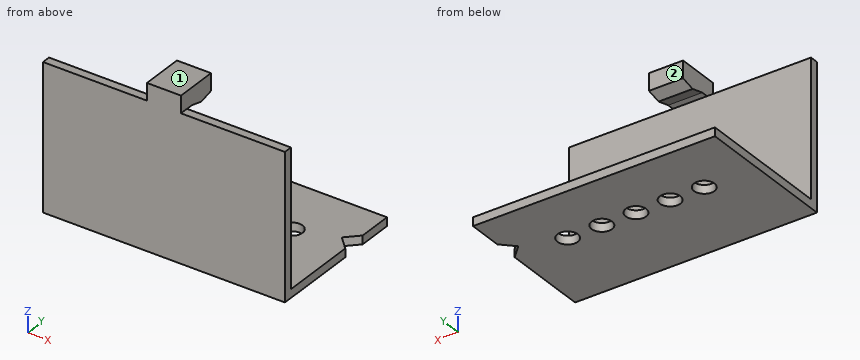
Autodesk Inventor part; units mm, degrees
ref_plane "YZ Plane" through (0, 0, 0) normal (1, 0, 0) x (0, 1, 0)
ref_plane "XZ Plane" through (0, 0, 0) normal (0, 1, 0) x (-1, 0, 0)
ref_plane "XY Plane" through (0, 0, 0) normal (0, 0, 1) x (1, 0, 0)
sketch "Sketch1" plane through (0, 0, 0) normal (0, 1, 0) x (-1, 0, 0)
  line L0 (45.085, 26.9875) -> (-45.085, 26.9875)
  line L1 (-45.085, 26.9875) -> (-45.085, -26.9875)
  line L2 (-45.085, -26.9875) -> (45.085, -26.9875)
  line L3 (45.085, -26.9875) -> (45.085, 26.9875)
  point P0 (0, 0)
  dimension "d0" = 90.17
  dimension "d1" = 45.085
  dimension "d2" = 53.975
  dimension "d3" = 26.9875
extrude "Extrusion1" add sketch "Sketch1" along normal blind 53.975
sketch "Sketch2" plane through (45.085, 0, 26.9875) normal (1, 0, 0) x (0, 0, -1)
  line L0 (0, 53.975) -> (53.975, 53.975)
  line L1 (0, 53.975) -> (50.8, 53.975)
  line L2 (50.8, 53.975) -> (50.8, 3.175)
  line L3 (50.8, 3.175) -> (0, 3.175)
  line L4 (0, 3.175) -> (0, 53.975)
  line L5 (0, 0) -> (53.975, 0)
  line L6 (53.975, 0) -> (53.975, 53.975)
  point P0 (26.9875, 0)
  dimension "d6" = 3.175
  dimension "d7" = 3.175
extrude "Extrusion2" cut sketch "Sketch2" against normal through all
sketch "Sketch3" plane through (0, 0, 0) normal (0, -1, 0) x (1, 0, 0)
  line L0 (-6.35, 23.8125) -> (6.35, 23.8125)
  line L1 (6.35, 23.8125) -> (6.35, 33.3375)
  line L2 (6.35, 33.3375) -> (-6.35, 33.3375)
  line L3 (-6.35, 33.3375) -> (-6.35, 23.8125)
  line L4 (1.9102, 23.8125) -> (1.9102, 26.9875) construction
  line L5 (-45.085, 26.9875) -> (45.085, 26.9875)
  point P0 (0, 0)
  dimension "d10" = 12.7
  dimension "d11" = 9.525
  dimension "d12" = 3.175
  dimension "d13" = 6.35
extrude "Extrusion3" add sketch "Sketch3" against normal blind 15.875
sketch "Sketch4" plane through (6.35, 0, 33.3375) normal (1, 0, 0) x (0, 0, -1)
  line L0 (9.525, 3.175) -> (6.35, 3.175)
  line L1 (9.525, 3.175) -> (9.525, 15.875)
  line L2 (0, 15.875) -> (9.525, 15.875)
  line L3 (6.35, 0) -> (6.35, 3.175)
  line L4 (6.35, 3.175) -> (6.35, 5.715)
  line L5 (6.35, 5.715) -> (6.35, 15.875) construction
  line L6 (6.35, 5.715) -> (7.62, 10.795)
  line L7 (7.62, 10.795) -> (6.35, 15.875)
  point P0 (33.3375, 0)
  dimension "d19" = 1.27
  dimension "d20" = 10.16
extrude "Extrusion4" cut sketch "Sketch4" against normal blind 15.875
sketch "Sketch5" plane through (45.085, 0, -26.9875) normal (0, 0, -1) x (-1, 0, 0)
  line L0 (19.6342, 31.75) -> (32.3596, 31.75) construction
  line L1 (32.3596, 31.75) -> (45.085, 31.75) construction
  line L2 (45.085, 31.75) -> (57.8104, 31.75) construction
  line L3 (57.8104, 31.75) -> (70.5358, 31.75) construction
  circle A0 centre (19.6342, 31.75) radius 3.81
  circle A1 centre (32.3596, 31.75) radius 3.81
  circle A2 centre (45.085, 31.75) radius 3.81
  circle A3 centre (57.8104, 31.75) radius 3.81
  circle A4 centre (70.5358, 31.75) radius 3.81
  line L4 (19.6342, 31.75) -> (5.2747, 31.75) construction
  line L5 (70.5358, 31.75) -> (84.8953, 31.75) construction
  line L6 (0, 53.975) -> (90.17, 53.975)
  point P0 (45.085, 0)
  point P1 (86.995, 3.175)
  point P2 (3.175, 3.175)
  dimension "d23" = 12.7254
  dimension "d24" = 7.62
  dimension "d26" = 22.225
extrude "Extrusion5" cut sketch "Sketch5" against normal blind 15.875
sketch "Sketch6" plane through (45.085, 3.175, -23.8125) normal (0, 0, 1) x (1, 0, 0)
  line L0 (0, 37.8968) -> (-4.572, 33.3248)
  line L1 (-4.572, 33.3248) -> (0, 28.7528)
  line L2 (0, 50.8) -> (-90.17, 50.8)
  line L3 (0, 37.8968) -> (0, 50.8)
  line L4 (0, 28.7528) -> (0, 25.3386)
  line L5 (0, 50.8) -> (0, 0)
  point P0 (-45.085, -3.175)
  dimension "d31" = 12.9032
  dimension "d32" = 45
  dimension "d33" = 45
  dimension "d35" = 4.572
extrude "Extrusion6" cut sketch "Sketch6" against normal blind 25.4
properties part number "PCB_Case02B"
For this review, take the finished solid that the model builds, in its own axes (mm). Face numbers are marked on the shaded views. A direction names the side the tool comes from. Round coordinates to 2 decimals unless told otherwise and drop trailing zeros. Order: outer loops, then holes, each group sorted by start corner. A loop starts at its lowest first (then second) coordinate and runs counter-clockwise, first axis right, second up. Notation, with made-up numbers: M 76,42.5 L 115,42.5 A29 cw 115,72.5 Z; hole C 9.5,68 d7. An arc over 180 degrees is marked long. Use a Markdown table: item, result. Add a question column.
Item 1: To check wall thickness, follow line 1 along X through (y, z) = (31, -25) (3 decimals); line 2 along Y through (x, z) = (0, -25.5) (3 decimals); line 3 along Z through (x, y) = (-11.5, 7). State the ranges of each line that lie inside material, in increasing order.
Item 2: Add section D-D, the plane z = 29. Give the boundary of the cut face in (x, y) (3 decimals), then the cut area to 3 significant figures.
Item 3: Insertion check: pin 1 (12 mm diameter, centred on x = 14, z = -18, fed in from +Y) (3 decimals); pin 2 (2 mm diameter, centred on x = -3.5, y = 20, fed in from +Z); pin 3 (6 mm diameter, centred on x = 12.73, y = 31.75, fed in from +Z) (3 decimals); pin 4 (4 mm diameter, centred on y = 5, z = 29, fed in from -X). Each pin has a flat end and moves straight along its axis. Give the tip position at first contact, or say it passes through.
Item 4: Add section B-B, the plane x = 0. Give the boundary of the cut face in (y, z) (1 decimal), then the cut area to 3 significant figures.
Item 5: Add section C-C, the plane y = 29.5. Give the boundary of the cut face in (x, z) (1 decimal).
Item 6: Tool access review of the marked faces 1 and 2: name each direction out of +Z, -Z, +X, -X, +Y, -Y from which nothing blocks a thin tool from reaching the whole face with its end or side.
Geometry results:
| question | item | result |
|---|---|---|
| 1 | line 1 | x = -45.085 to -29.186, -21.715 to -16.461, -8.99 to -3.735, 3.735 to 8.99, 16.461 to 21.715, 29.186 to 45.085 |
| 1 | line 2 | y = 0 to 27.94, 35.56 to 53.975 |
| 1 | line 3 | z = -26.99 to -23.81 |
| 2 | outline | M -6.35,0 L 6.35,0 L 6.35,15.875 L -6.35,15.875 Z |
| 2 | area | 202 mm² |
| 3 | pin 1 | stops at y = 53.975 |
| 3 | pin 2 | stops at z = -23.81 |
| 3 | pin 3 | passes through |
| 3 | pin 4 | stops at x = -6.35 |
| 4 | outline | M 0,-27 L 27.9,-27 L 27.9,-23.8 L 3.2,-23.8 L 3.2,27 L 5.7,27 L 10.8,25.7 L 15.9,27 L 15.9,33.3 L 0,33.3 Z; M 35.6,-27 L 54,-27 L 54,-23.8 L 35.6,-23.8 Z |
| 4 | area | 416 mm² |
| 5 | outline | M -45.1,-27 L -28.5,-27 L -28.5,-23.8 L -45.1,-23.8 Z; M -22.4,-27 L -15.8,-27 L -15.8,-23.8 L -22.4,-23.8 Z; M -9.7,-27 L -3.1,-27 L -3.1,-23.8 L -9.7,-23.8 Z; M 3.1,-27 L 9.7,-27 L 9.7,-23.8 L 3.1,-23.8 Z; M 15.8,-27 L 22.4,-27 L 22.4,-23.8 L 15.8,-23.8 Z; M 28.5,-27 L 45.1,-27 L 45.1,-23.8 L 28.5,-23.8 Z |
| 6 | face 1 | +Z, +X, -X, +Y, -Y |
| 6 | face 2 | +Z, +X, -X, +Y |
